```python
from build123d import *

# Parameters (mm, degrees)
SKETCH_R             = 1.75
SKETCH_R_2           = 2.75
PAD_DEPTH            = 8
PAD001_DEPTH         = 20
SKETCH004_R          = 2.75
POCKET_DEPTH         = 23.001
SKETCH005_R          = 2.75
POCKET001_DEPTH      = 20.001
POCKET001_DEPTH_BACK = 8.001
SKETCH008_R          = 4
SKETCH008_R_2        = 2.75
PAD005_DEPTH         = 2
SKETCH009_R          = 3.5
SKETCH009_R_2        = 2.75
PAD006_DEPTH         = 0.55
SKETCH010_R          = 4
SKETCH010_R_2        = 2.75
PAD007_DEPTH         = 12.1
SKETCH011_R          = 3.5
SKETCH011_R_2        = 2.75
PAD008_DEPTH         = 0.55
POCKET004_DEPTH      = 2
SKETCH020_W          = 4
SKETCH020_H          = 10.5
PAD013_DEPTH         = 33.4
PAD013_DEPTH_BACK    = 23
SKETCH021_W          = 27
SKETCH021_H          = 5
PAD014_DEPTH         = 3
SKETCH023_R          = 3.75
POCKET007_DEPTH      = 1


with BuildPart() as part:
    # Sketch → Pad (new body)
    with BuildSketch(Plane.XY):
        Polygon((0, 23), (73, 23), (73, -3.2), (65, -3.2), (65, -33.4), (0, -33.4), (-2, -33.4), (-2, 23), align=None)
        with Locations((3.5, 10.3)):
            Circle(SKETCH_R, mode=Mode.SUBTRACT)
        with Locations((23.5, 10.3)):
            Circle(SKETCH_R, mode=Mode.SUBTRACT)
        with Locations((3.5, -9.7)):
            Circle(SKETCH_R, mode=Mode.SUBTRACT)
        with Locations((23.5, -9.7)):
            Circle(SKETCH_R, mode=Mode.SUBTRACT)
        with Locations((55, 7)):
            Circle(SKETCH_R_2, mode=Mode.SUBTRACT)
        with Locations((41.5, -15)):
            Circle(SKETCH_R_2, mode=Mode.SUBTRACT)
        with Locations((54.45, -27.95)):
            Circle(SKETCH_R_2, mode=Mode.SUBTRACT)
        with Locations((66, 7)):
            Circle(SKETCH_R_2, mode=Mode.SUBTRACT)
    extrude(amount=PAD_DEPTH)

    # Sketch001 → Pad001 (join)
    with BuildSketch(Plane(origin=(0, 0, 0), x_dir=(1, 0, 0), z_dir=(0, 0, -1))):
        Polygon((73, -23), (39.5, -23), (39.5, 3), (46.5, 3), (57, 16.2), (65, 16.2), (65, 3.2), (47.5, 3.2), (47.5, -17), (73, -17), align=None)
    extrude(amount=PAD001_DEPTH)

    # Sketch004 → Pocket (cut, through all)
    with BuildSketch(Plane.XZ):
        with Locations((55, -10)):
            Circle(SKETCH004_R)
        with Locations((66, -10)):
            Circle(SKETCH004_R)
    extrude(amount=-POCKET_DEPTH, mode=Mode.SUBTRACT)

    # Sketch005 → Pocket001 (cut, two sides)
    with BuildSketch(Plane.XY) as pocket001_sk:
        with Locations((58, -9.7)):
            Circle(SKETCH005_R)
        with Locations((43, 7)):
            Circle(SKETCH005_R)
    extrude(amount=-POCKET001_DEPTH, mode=Mode.SUBTRACT)
    extrude(pocket001_sk.sketch, amount=POCKET001_DEPTH_BACK, mode=Mode.SUBTRACT)

    # Sketch008 → Pad005 (join)
    with BuildSketch(Plane.XY):
        with Locations((41.5, -15)):
            Circle(SKETCH008_R)
        with Locations((41.5, -15)):
            Circle(SKETCH008_R_2, mode=Mode.SUBTRACT)
    extrude(amount=-PAD005_DEPTH)

    # Sketch009 (on Face30 of Pad005) → Pad006 (join)
    with BuildSketch(Plane(origin=(0, 0, -2), x_dir=(1, 0, 0), z_dir=(0, 0, -1))):
        with Locations((41.5, 15)):
            Circle(SKETCH009_R)
        with Locations((41.5, 15)):
            Circle(SKETCH009_R_2, mode=Mode.SUBTRACT)
    extrude(amount=PAD006_DEPTH)

    # Sketch010 → Pad007 (join)
    with BuildSketch(Plane.XY):
        with Locations((54.45, -27.95)):
            Circle(SKETCH010_R)
        with Locations((54.45, -27.95)):
            Circle(SKETCH010_R_2, mode=Mode.SUBTRACT)
    extrude(amount=-PAD007_DEPTH)

    # Sketch011 (on Face32 of Pad007) → Pad008 (join)
    with BuildSketch(Plane(origin=(0, 0, -12.1), x_dir=(1, 0, 0), z_dir=(0, 0, -1))):
        with Locations((54.45, 27.95)):
            Circle(SKETCH011_R)
        with Locations((54.45, 27.95)):
            Circle(SKETCH011_R_2, mode=Mode.SUBTRACT)
    extrude(amount=PAD008_DEPTH)

    # Sketch017 (on DatumPlane) → Pocket004 (cut)
    with BuildSketch(Plane.XY.offset(8)):
        with BuildLine():
            ThreePointArc((55, 13), (49, 7), (55, 1))
            Line((55, 1), (66, 1))
            ThreePointArc((66, 1), (72, 7), (66, 13))
            Line((66, 13), (55, 13))
        make_face()
    extrude(amount=-POCKET004_DEPTH, mode=Mode.SUBTRACT)

    # Sketch020 → Pad013 (join, two sides)
    with BuildSketch(Plane.XZ) as pad013_sk:
        with Locations((29, -5.25)):
            Rectangle(SKETCH020_W, SKETCH020_H)
    extrude(amount=PAD013_DEPTH)
    extrude(pad013_sk.sketch, amount=-PAD013_DEPTH_BACK)

    # Sketch021 → Pad014 (join)
    with BuildSketch(Plane(origin=(0, 0, 0), x_dir=(-1, 0, 0), z_dir=(0, 0, -1))):
        with Locations((-13.5, -24.9)):
            Rectangle(SKETCH021_W, SKETCH021_H)
    extrude(amount=PAD014_DEPTH)

    # Sketch023 (on DatumPlane) → Pocket007 (cut)
    with BuildSketch(Plane.XY.offset(8)):
        with Locations((3.5, 10.3)):
            Circle(SKETCH023_R)
        with Locations((23.5, 10.3)):
            Circle(SKETCH023_R)
        with Locations((3.5, -9.7)):
            Circle(SKETCH023_R)
        with Locations((23.5, -9.7)):
            Circle(SKETCH023_R)
    extrude(amount=-POCKET007_DEPTH, mode=Mode.SUBTRACT)


solid = part.part
```
Part model, mm, in its own coordinate system. A direction names the side the tool comes from. Round coordinates to 2 decimals unless told otherwise and drop trailing zeros. Write each loop counter-clockwise with the first axis right and the second up, starting at its lowest first coordinate (ties: lowest second). Pieces come first, ordered by that corner, then holes. Notation, with made-up numbers: (72.5, -22.5) -> (76.5, -22.5) arc R18 ccw to (76.5, -7.5) -> close; hole circle Ø9 at (88.25, -24.5). An arc over 180 degrees is marked (long way). Return JSON: item names as keys, results as strings. Group by question number.
Q1. Pin check, flat tips, straight feed: pin 1 (9 mm diameter, centred on x = 66, z = -10, fed in from -Y); pin 2 (8 mm diameter, centred on y = -3, z = -12.5, fed in from +X); pin 3 (2 mm diameter, centred on x = 42.5, z = -5.5, fed in from -Y); pin 4 (2 mm diameter, centred on x = 23.5, y = 10.3, fed in from -Z). Stop position of each tip, or through.
Q2. Mould opens along Y. For faces 5 (the flat face through (65, -15, -3)), 6 (the flat face through (31, -33.4, 3)), 7 (the cylindrical face through (22.21, -8.52, 3.45)) say: pulls with the +Y half, pulls with the -Y half, needs draft (parallel to the pull), parting line crosses it, or undercut.
Q3. Saw through at C-C on z = -16.75. Write the cut outline in (x, y).
Q4. Saw through at B-B on x = 3.5. Write the cut outline in (y, z), plus the area to 3 significant figures.
Q5. Saw through at A-A on z = 4.25. State how many separate pieces and enclosed holes the cut face has, plus the area to 3 significant figures.
Q6. Probe L1, parallel to X at y = 7, z = 1.5; L2, parallel to Y at x = 3.5, z = 4; L3, parallel to X at y = 10.3, z = 3.5. List the from-to ranges inside material, lowest first. Write a range as [from, to].
Q7. Which spindle directions (+Z, -Z, +X, -X, +Y, -Y) get a long thin tool onto all of the face, cutting with end or side? Do faces 1 (the flat face through (69, -3.2, 4)), 2 (the flat face through (56, -3.2, -10)), 3 (the cylindrical face through (58.265, -26.749, -5.965)), 4 (the cylindrical face through (25.23, 6.973, 7.507)). Say none if no direction does.
Q8. Saw through at D-D on y = -15. Write the cut outline in (x, z).
Answer:
{
 "1": {"pin 1": "y = -16.2", "pin 2": "x = 65", "pin 3": "y = -3", "pin 4": "through"},
 "2": {"face 5": "needs draft", "face 6": "pulls with the -Y half", "face 7": "undercut"},
 "3": {"outline": "(39.5, -3) -> (46.5, -3) -> (57, -16.2) -> (65, -16.2) -> (65, -3.2) -> (47.5, -3.2) -> (47.5, 17) -> (73, 17) -> (73, 23) -> (39.5, 23) -> close; hole circle Ø5.5 at (43, 7); hole circle Ø5.5 at (58, -9.7)"},
 "4": {"outline": "(-33.4, 0) -> (-27.4, 0) -> (-27.4, -3) -> (-22.4, -3) -> (-22.4, 0) -> (-11.45, 0) -> (-11.45, 7) -> (-13.45, 7) -> (-13.45, 8) -> (-33.4, 8) -> close; (-7.95, 0) -> (8.55, 0) -> (8.55, 7) -> (6.55, 7) -> (6.55, 8) -> (-5.95, 8) -> (-5.95, 7) -> (-7.95, 7) -> close; (12.05, 0) -> (23, 0) -> (23, 8) -> (14.05, 8) -> (14.05, 7) -> (12.05, 7) -> close", "area": "402 mm2"},
 "5": {"separate pieces": "1", "enclosed holes": "10", "area": "3,810 mm2"},
 "6": {"L1": "[-2, 40.25], [45.75, 52.25], [57.75, 63.25], [68.75, 73]", "L2": "[-33.4, -11.45], [-7.95, 8.55], [12.05, 23]", "L3": "[-2, 1.75], [5.25, 21.75], [25.25, 73]"},
 "7": {"face 1": "+Z, -Z, +X, -Y", "face 2": "-Z, +X", "face 3": "-Z", "face 4": "+Z"},
 "8": {"outline": "(-2, 0) -> (27, 0) -> (27, -10.5) -> (31, -10.5) -> (31, 0) -> (37.5, 0) -> (37.5, -2) -> (38, -2) -> (38, -2.55) -> (38.75, -2.55) -> (38.75, 8) -> (-2, 8) -> close; (44.25, -2.55) -> (45, -2.55) -> (45, -2) -> (45.5, -2) -> (45.5, 0) -> (56.05, 0) -> (56.05, -20) -> (65, -20) -> (65, 8) -> (44.25, 8) -> close"}
}
